Source: CAD feature listing. Evaluate the final solid. Frame: model axes, mm. Coordinates: 2 decimals unless noted, no trailing zeros. Loops run counter-clockwise (first coordinate to the right, second up) from the corner with the lowest first, then second, coordinate; pieces in that order, holes last.
Item 1: Section query C-C, the plane y = -7.65. Return the cut outline in (x, z) (3 decimals).
Item 2: Section query A-A, the plane x = 35. Return the cut outline in (y, z), then the cut area to 3 significant figures.
Item 3: Section query B-B, the plane x = 47. Return the cut outline in (y, z).
Item 4: Line query: probe 1 along Y at (x, z) = (25, -0.55); probe 2 along X at (y, z) = (24, -0.2); probe 3 along X at (y, z) = (-8, -0.35). Output: solid intervals per line, ascending.
Item 5: Pull-direction query (Y, two-part tool) for faces 1 (the cylindrical face through (-36.281, 24.364, -0.789)), 2 (the flat face through (-1, 0, 0)); classes: +Y half, -Y half, draft (parallel to the pull), parting line (faces both ways), or undercut.
```python
from build123d import *

# Parameters (mm, degrees)
F0_W     = 100
F0_H     = 60
F0_R     = 1.5
F0_R_2   = 1.6
F0_H_2   = 1
F1_DEPTH = 1.6


with BuildPart() as f1:
    # F0 (on Top) → F1 (new body)
    with BuildSketch(Plane.XY):
        Rectangle(F0_W, F0_H)
        with Locations((-47, -27)):
            Circle(F0_R, mode=Mode.SUBTRACT)
        with Locations((-35.175, -7.65)):
            Circle(F0_R, mode=Mode.SUBTRACT)
        with Locations((15, -25)):
            Circle(F0_R_2, mode=Mode.SUBTRACT)
        with Locations((25, -25)):
            Circle(F0_R_2, mode=Mode.SUBTRACT)
        with Locations((35, -25)):
            Circle(F0_R_2, mode=Mode.SUBTRACT)
        with Locations((47, -27)):
            Circle(F0_R, mode=Mode.SUBTRACT)
        with Locations((25, -15)):
            Circle(F0_R_2, mode=Mode.SUBTRACT)
        with Locations((39.825, -7.65)):
            Circle(F0_R, mode=Mode.SUBTRACT)
        with Locations((-47, 27)):
            Circle(F0_R, mode=Mode.SUBTRACT)
        with Locations((-35.175, 23.35)):
            Circle(F0_R, mode=Mode.SUBTRACT)
        with Locations((39.825, 23.35)):
            Circle(F0_R, mode=Mode.SUBTRACT)
        with Locations((47, 27)):
            Circle(F0_R, mode=Mode.SUBTRACT)
        with Locations((0, -30.5)):
            Rectangle(F0_W, F0_H_2)
    extrude(amount=-F1_DEPTH)


solid = f1.part
```
Verdict:
1. outline: (-50, -1.6) - (-36.675, -1.6) - (-36.675, 0) - (-50, 0) - close; (-33.675, -1.6) - (38.325, -1.6) - (38.325, 0) - (-33.675, 0) - close; (41.325, -1.6) - (50, -1.6) - (50, 0) - (41.325, 0) - close
2. outline: (-31, -1.6) - (-26.6, -1.6) - (-26.6, 0) - (-31, 0) - close; (-23.4, -1.6) - (30, -1.6) - (30, 0) - (-23.4, 0) - close
2. area: 92.5 mm2
3. outline: (-31, -1.6) - (-28.5, -1.6) - (-28.5, 0) - (-31, 0) - close; (-25.5, -1.6) - (25.5, -1.6) - (25.5, 0) - (-25.5, 0) - close; (28.5, -1.6) - (30, -1.6) - (30, 0) - (28.5, 0) - close
4. probe 1: y = -31 to -26.6, -23.4 to -16.6, -13.4 to 30
4. probe 2: x = -50 to -36.53, -33.82 to 38.47, 41.18 to 50
4. probe 3: x = -50 to -36.63, -33.72 to 38.37, 41.28 to 50
5. face 1: undercut
5. face 2: draft
